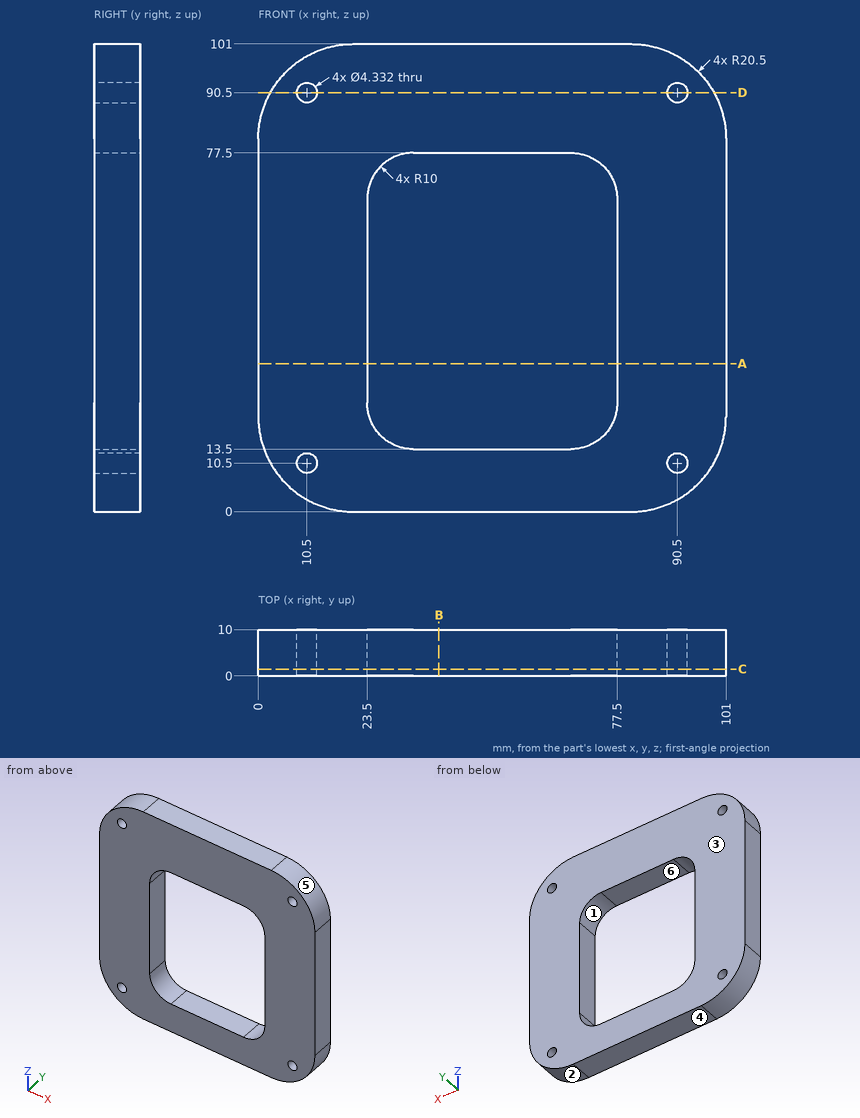
Print and shaded views of the part. All mm, measured from the part's lowest x, y and z. A direction names the side the tool comes from. Coordinates: 2 decimals unless noted, no trailing zeros. Loops run counter-clockwise (first coordinate to the right, second up) from the corner with the lowest first, then second, coordinate; pieces in that order, holes last. Notation, with made-up numbers: (60.25, 32.5) - (108.25, 32.5) arc R26 ccw to (108.25, 54.5) - close; hole circle Ø7 at (84.5, -0.5). An arc over 180 degrees is marked (long way). Write item = value, one per line. Start each with the question number.
Item 1: Cut at C-C, the plane y = 1.5. Give the cut face in (x, z).
Item 2: Cut at D-D, the plane z = 90.5. Give the cut face in (x, y), and give its area (3 significant figures).
Item 3: Wall check: L1, parallel to X at y = 5.5, z = 91; L2, parallel to X at y = 9, z = 51.5; L3, parallel to X at y = 4, z = 10.5. Give the ranges that are in metal, low to high. Write a range as from..to.
Item 4: Cut at A-A, the plane z = 32. Give the cut face in (x, y), and give its area (3 significant figures).
Item 5: 3-axis set-ups, long thin cutter, end or side, ignore diameter. For the marked faces 1 and 2: which of +Z, -Z, +X, -X, +Y, -Y reach the whole face in a straight line?
Item 6: Mould opens along Z. For the marked faces 3, 4, 5 and 6 say: released by +Z, released by -Z, zero draft, split by the parting line, or undercut.
Item 7: Cut at B-B, the plane x = 39. Give the cut face in (y, z), and give its area (3 significant figures).
Item 8: Flat gauge pins, fed straight in: pin 1 Ø5 at (x, y) = (61, 3) entering from -Z; pin 2 Ø4 at (x, z) = (10.5, 10.5) entering from -Y. Where does each tip first touch, or does it go through?
The answers:
q1.outline = (0, 20.5) arc R20.5 ccw to (20.5, 0) - (80.5, 0) arc R20.5 ccw to (101, 20.5) - (101, 80.5) arc R20.5 ccw to (80.5, 101) - (20.5, 101) arc R20.5 ccw to (0, 80.5) - close; hole circle Ø4.33 at (10.5, 10.5); hole circle Ø4.33 at (10.5, 90.5); hole (23.5, 23.5) arc R10 ccw to (33.5, 13.5) - (67.5, 13.5) arc R10 ccw to (77.5, 23.5) - (77.5, 67.5) arc R10 ccw to (67.5, 77.5) - (33.5, 77.5) arc R10 ccw to (23.5, 67.5) - close; hole circle Ø4.33 at (90.5, 10.5); hole circle Ø4.33 at (90.5, 90.5)
q2.outline = (2.6, 0) - (8.33, 0) - (8.33, 10) - (2.6, 10) - close; (12.67, 0) - (88.33, 0) - (88.33, 10) - (12.67, 10) - close; (92.67, 0) - (98.4, 0) - (98.4, 10) - (92.67, 10) - close
q2.area = 871 mm2
q3.L1 = 2.89..8.39, 12.61..88.39, 92.61..98.11
q3.L2 = 0..23.5, 77.5..101
q3.L3 = 2.6..8.33, 12.67..88.33, 92.67..98.4
q4.outline = (0, 0) - (23.5, 0) - (23.5, 10) - (0, 10) - close; (77.5, 0) - (101, 0) - (101, 10) - (77.5, 10) - close
q4.area = 470 mm2
q5.face_1 = +Y, -Y
q5.face_2 = -Z, +X, +Y, -Y
q6.face_3 = zero draft
q6.face_4 = released by -Z
q6.face_5 = released by +Z
q6.face_6 = undercut
q7.outline = (0, 0) - (10, 0) - (10, 13.5) - (0, 13.5) - close; (0, 77.5) - (10, 77.5) - (10, 101) - (0, 101) - close
q7.area = 370 mm2
q8.pin_1 = 0
q8.pin_2 = through
